Read the model definition and answer for the solid it produces. Units are mm, in the model's axes. A direction names the side the tool comes from. Coordinates: 2 decimals unless noted, no trailing zeros. Write each loop counter-clockwise with the first axis right and the second up, starting at its lowest first coordinate (ties: lowest second). Pieces come first, ordered by that corner, then holes.
(1) The part is cut by section A-A, the plane x = 22. Determine the outline of the cut face in (y, z).
(2) Which of the six approach directions +Z, -Z, +X, -X, +Y, -Y give full straight-line access (tool end or side, diameter ignored) to faces 4 (the flat face through (-5.08, 8, 43)), 5 (the cylindrical face through (10.09, 8.67, -52.55)), 6 (the conical face through (15.4, 8.72, -52.4)), 7 (the flat face through (50, 13, -63.5)), 8 (the cylindrical face through (51.26, 0.56, -70.43))?
(3) The part is cut by section C-C, the plane z = -55.88. State how many separate pieces and enclosed holes the cut face has, and give its area (3 significant figures).
(4) Given pin 1 (10 mm diameter, centred on x = -10, z = 40.5, fed in from -Y); pin 2 (4 mm diameter, centred on y = 7.62, z = 55.88, fed in from -X), each flat-ended and moving along its own axis, determine where each tip first touches the part or whether it passes through.
(5) Determine the mould class of faces 1 (the flat face through (-50, 8, -76.2)), 2 (the cylindrical face through (51.26, 0.56, 70.43)), 3 (the flat face through (96.52, 8, 1)) for opening direction X: pulls with the +X half, pulls with the -X half, needs draft (parallel to the pull), parting line crosses it, or undercut.
(6) Straight lines are drawn through the part: line 1 along X through (y, z) = (9.5, 0); line 2 along X through (y, z) = (3, 8.5); line 3 along Z through (x, y) = (-88.75, 7.62). For each, find the intervals that lie inside material, in ascending order.
(7) The part is cut by section B-B, the plane z = -31. Determine the outline of the cut face in (x, y), and give its area (3 significant figures).
(8) The part is cut by section D-D, the plane x = -58. Determine the outline of the cut face in (y, z), and give its area (3 significant figures).
```python
from build123d import *

# Parameters (mm, degrees)
SKETCH3_R           = 10.16
SKETCH3_R_2         = 5.08
SKETCH3_W           = 91.44
SKETCH3_H           = 152.4
SKETCH3_W_2         = 66.04
SKETCH3_H_2         = 127
BOSS_EXTRUDE1_DEPTH = 15.24
CUT_EXTRUDE1_REACH  = 122
SKETCH4_R           = 3.4925
CHAMFER1_SIZE       = 6.604
CHAMFER1_SIZE2      = 9.431489437
CHAMFER2_SIZE       = 2.54
FILLET1_R           = 5.08
SKETCH5_RX          = 0.7366
SKETCH5_RY          = 0.736599138
CUT_EXTRUDE2_DEPTH  = 12.7
SKETCH6_R           = 1.015962928
SKETCH6_RX          = 0.7366
SKETCH6_RY          = 0.736573123
CUT_EXTRUDE3_DEPTH  = 12.7


with BuildPart() as part:
    # Sketch3 → Boss-Extrude1 (new body)
    # profile 1 of 2: a face of its own
    with BuildSketch(Plane(origin=(0, 0, 0), x_dir=(1, 0, 0), z_dir=(0, 1, 0))):
        Circle(SKETCH3_R)
        with Locations(Location((0, 0, 0), (0, 0, 90))):
            Circle(SKETCH3_R_2, mode=Mode.SUBTRACT)
    # profile 2 of 2: a face of its own
    with BuildSketch(Plane(origin=(0, 0, 0), x_dir=(1, 0, 0), z_dir=(0, 1, 0))):
        with Locations((50.8, 0)):
            Rectangle(SKETCH3_W, SKETCH3_H)
        with Locations((50.8, 0)):
            Rectangle(SKETCH3_W_2, SKETCH3_H_2, mode=Mode.SUBTRACT)
    boss_extrude1 = extrude(amount=BOSS_EXTRUDE1_DEPTH)

    # Cut-Extrude1: up to this face of the body (flat: up to its plane)
    cut_extrude1_end = Plane(part.part.faces().sort_by_distance((96.52, 7.62, 0))[0])
    # Sketch4 → Cut-Extrude1 (cut, up to the picked face)
    with BuildSketch(Plane.ZY.offset(-5.08), mode=Mode.PRIVATE) as cut_extrude1_sk1:
        with Locations((-55.88, 7.62)):
            Circle(SKETCH4_R)
    cut_extrude1_tool1 = split(extrude(cut_extrude1_sk1.sketch, amount=-CUT_EXTRUDE1_REACH, mode=Mode.PRIVATE), bisect_by=cut_extrude1_end, keep=Keep.BOTH, mode=Mode.PRIVATE)
    # Sketch4 → Cut-Extrude1 (cut, up to the picked face)
    with BuildSketch(Plane.ZY.offset(-5.08), mode=Mode.PRIVATE) as cut_extrude1_sk2:
        with Locations((55.88, 7.62)):
            Circle(SKETCH4_R)
    cut_extrude1_tool2 = split(extrude(cut_extrude1_sk2.sketch, amount=-CUT_EXTRUDE1_REACH, mode=Mode.PRIVATE), bisect_by=cut_extrude1_end, keep=Keep.BOTH, mode=Mode.PRIVATE)
    cut_extrude1_1 = cut_extrude1_tool1.solids().sort_by(Axis((5.08, 7.62, -55.88), (1, 0, 0)))[0]
    add(cut_extrude1_1, mode=Mode.SUBTRACT)
    cut_extrude1_2 = cut_extrude1_tool2.solids().sort_by(Axis((5.08, 7.62, 55.88), (1, 0, 0)))[0]
    add(cut_extrude1_2, mode=Mode.SUBTRACT)
    cut_extrude1 = cut_extrude1_1 + cut_extrude1_2  # Cut-Extrude1 as one shape, for the pattern or mirror that repeats it

    # Chamfer1
    chamfer1_edges = [part.edges().sort_by_distance(p)[0] for p in [
        (50.8, 0, -63.5),
        (50.8, 0, 63.5),
    ]]
    chamfer1_side = [part.faces().sort_by_distance(p)[0] for p in [
        (94.659720924, 0, 0),
    ]]
    chamfer(chamfer1_edges, length=CHAMFER1_SIZE, length2=CHAMFER1_SIZE2, reference=chamfer1_side[0])

    # Chamfer2
    chamfer2_edges = [part.edges().sort_by_distance(p)[0] for p in [
        (96.52, 7.62, -59.3725),
        (17.78, 7.62, -59.3725),
        (96.52, 7.62, 52.3875),
        (17.78, 7.62, 52.3875),
    ]]
    chamfer(chamfer2_edges, length=CHAMFER2_SIZE)

    # Fillet1
    fillet1_edges = [part.edges().sort_by_distance(p)[0] for p in [
        (50.8, 9.431489437, 63.5),
        (50.8, 0, -70.104),
        (50.8, 0, 70.104),
        (50.8, 9.431489437, -63.5),
    ]]
    fillet(fillet1_edges, radius=FILLET1_R)

    # Sketch5 → Cut-Extrude2 (cut)
    with BuildSketch(Plane.XY.offset(-63.5)):
        with BuildLine():
            ThreePointArc((47.502994006, 11.033207367), (47.953744135, 11.407651091), (48.122732414, 11.968745328))
            ThreePointArc((48.122732414, 11.968745328), (47.473130673, 12.916377519), (46.355000482, 12.652229708))
            ThreePointArc((46.355000482, 12.652229708), (46.090734793, 11.968745328), (46.355000482, 11.285260949))
            ThreePointArc((46.355000482, 11.285260949), (46.519064449, 11.139951899), (46.710473201, 11.033207367))
            Line((46.710473165, 11.033207284), (47.502994041, 11.033207284))
        make_face()
        with BuildLine():
            ThreePointArc((46.710473201, 11.033207367), (47.106733603, 10.952746518), (47.502994006, 11.033207367))
            Line((47.502994041, 11.033207284), (46.710473165, 11.033207284))
        make_face()
        with Locations(Location((54.472733603, 11.968745328), (0, 0, -180))):
            Ellipse(SKETCH5_RX, SKETCH5_RY)
    extrude(amount=-CUT_EXTRUDE2_DEPTH, mode=Mode.SUBTRACT)

    # Sketch6 → Cut-Extrude3 (cut)
    with BuildSketch(Plane(origin=(0, 0, 63.5), x_dir=(-1, 0, 0), z_dir=(0, 0, -1))):
        with Locations((-54.493266397, 12.147267432)):
            Circle(SKETCH6_R)
        with Locations(Location((-47.127266397, 12.147267432), (0, 0, 0))):
            Ellipse(SKETCH6_RX, SKETCH6_RY)
    extrude(amount=-CUT_EXTRUDE3_DEPTH, mode=Mode.SUBTRACT)

    # Mirror1: Boss-Extrude1, Cut-Extrude1 across plane
    add(boss_extrude1.mirror(Plane(origin=(0, 0, 0), x_dir=(0, 0, 1), z_dir=(1, 0, 0))))
    add(cut_extrude1.mirror(Plane(origin=(0, 0, 0), x_dir=(0, 0, 1), z_dir=(1, 0, 0))), mode=Mode.SUBTRACT)


solid = part.part
```
Computed:
1. outline: (0, -76.2) - (15.24, -76.2) - (15.24, -63.5) - (11.03, -63.5) arc R5.08 ccw to (8.12, -64.42) - (2.17, -68.59) arc R5.08 ccw to (0, -72.75) - close; (0, 72.75) arc R5.08 ccw to (2.17, 68.59) - (8.12, 64.42) arc R5.08 ccw to (11.03, 63.5) - (15.24, 63.5) - (15.24, 76.2) - (0, 76.2) - close
2. face 4: +Z, +Y, -Y
2. face 5: +X, -X
2. face 6: none
2. face 7: +Y, -Y
2. face 8: -Y
3. separate pieces: 8
3. enclosed holes: 0
3. area: 406 mm2
4. pin 1: stops at y = 0
4. pin 2: passes through
5. face 1: needs draft
5. face 2: undercut
5. face 3: pulls with the +X half
6. line 1: x = -96.52 to -83.82, -17.78 to -5.08, 5.08 to 17.78, 83.82 to 96.52
6. line 2: x = -96.52 to -83.82, -17.78 to 17.78, 83.82 to 96.52
6. line 3: z = -76.2 to -59.37, -52.39 to 52.39, 59.37 to 76.2
7. outline: (-96.52, 0) - (-83.82, 0) - (-83.82, 15.24) - (-96.52, 15.24) - close; (-17.78, 0) - (-5.08, 0) - (-5.08, 15.24) - (-17.78, 15.24) - close; (5.08, 0) - (17.78, 0) - (17.78, 15.24) - (5.08, 15.24) - close; (83.82, 0) - (96.52, 0) - (96.52, 15.24) - (83.82, 15.24) - close
7. area: 774 mm2
8. outline: (0, -76.2) - (15.24, -76.2) - (15.24, -63.5) - (0, -63.5) - close; (0, 63.5) - (15.24, 63.5) - (15.24, 76.2) - (0, 76.2) - close
8. area: 387 mm2
